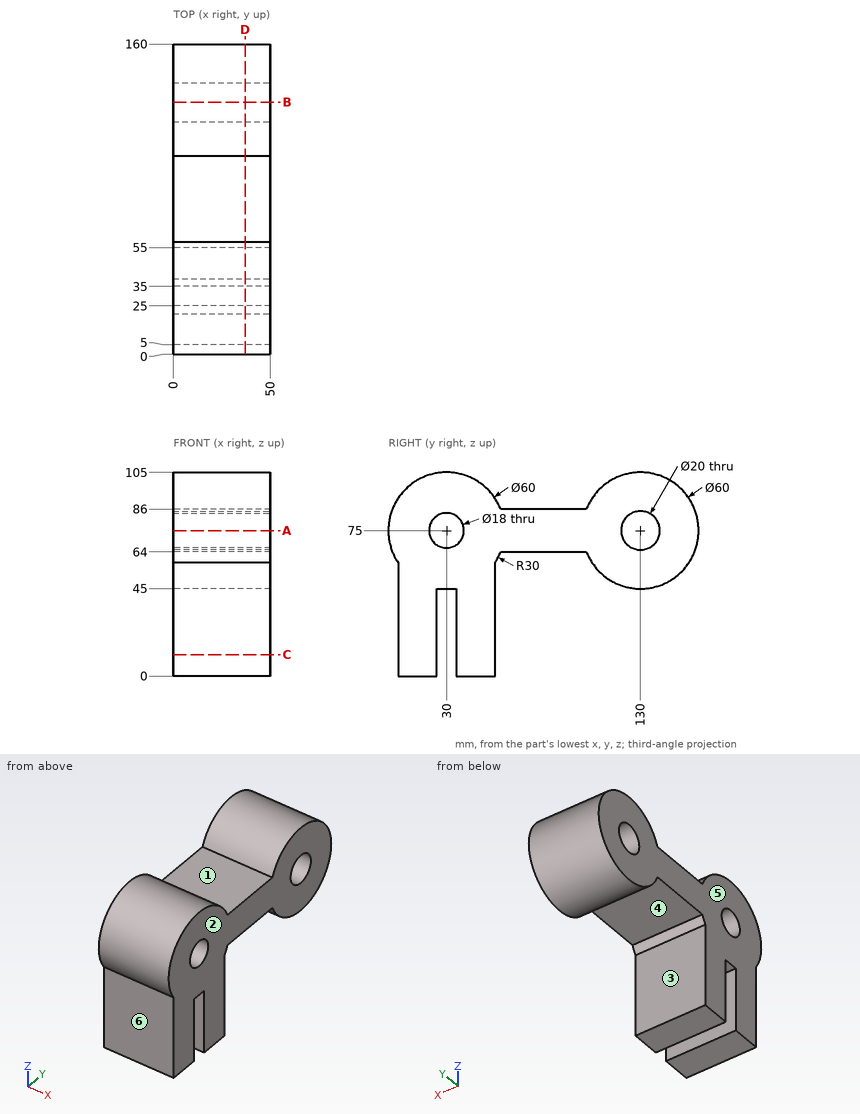
Print and shaded views of the part. All mm, measured from the part's lowest x, y and z. A direction names the side the tool comes from. Coordinates: 2 decimals unless noted, no trailing zeros. Loops run counter-clockwise (first coordinate to the right, second up) from the corner with the lowest first, then second, coordinate; pieces in that order, holes last. Notation, with made-up numbers: (5.5, -37) -> (41.5, -37) arc R24 cw to (41.5, -5) -> close; hole circle Ø6 at (46.5, -32.5). An arc over 180 degrees is marked (long way). Use a Markdown table: item, result. Add a question column.
Item 1: Band-saw the part on B-B on y = 130. Write the cut outline in (x, z).
Item 2: Probe probe 1 along Y at (x, z) = (18.5, 75); probe 2 along Y at (x, z) = (8.5, 41); probe 3 along Y at (x, z) = (46, 97.5). List the from-to ranges inside material, lowest first.
Item 3: Which spindle directions (+Z, -Z, +X, -X, +Y, -Y) get a long thin tool onto all of the face, cutting with end or side? Do the marked faces 1, 2 and 3. Say none if no direction does.
Item 4: Pull direction Y, two halves, no side cores. Call the marked faces 4, 5 and 6: +Y half, -Y half, draft (parallel to the pull), parting line (faces both ways), or undercut.
Item 5: Band-saw the part on A-A on z = 75. Write the cut outline in (x, y).
Item 6: Flat gauge pins, fed straight in: P1, Ø8, axis at y = 26.5, z = 15, coming from the -X side; P2, Ø2, axis at x = 22, y = 127.5, coming from the -Z side; P3, Ø16, axis at y = 30, z = 75, coming from the -X side; P4, Ø3, axis at x = 39, y = 84, coming from the +Z side. Where does each tip first touch, or does it go through?
Item 7: Band-saw the part on C-C on z = 11. Write the cut outline in (x, y), plus the area to 3 significant figures.
Item 8: Band-saw the part on D-D on x = 37. Write the cut outline in (y, z).
Geometry says:
| question | item | result |
|---|---|---|
| 1 | outline | (0, 45) -> (50, 45) -> (50, 65) -> (0, 65) -> close; (0, 85) -> (50, 85) -> (50, 105) -> (0, 105) -> close |
| 2 | probe 1 | 0 to 21, 39 to 120, 140 to 160 |
| 2 | probe 2 | 5 to 25, 35 to 55 |
| 2 | probe 3 | 10.16 to 49.84, 110.16 to 149.84 |
| 3 | face 1 | +Z, +X, -X |
| 3 | face 2 | +Z, -Z, +X, +Y, -Y |
| 3 | face 3 | -Z, +X, -X |
| 4 | face 4 | undercut |
| 4 | face 5 | draft |
| 4 | face 6 | -Y half |
| 5 | outline | (0, 0) -> (50, 0) -> (50, 21) -> (0, 21) -> close; (0, 39) -> (50, 39) -> (50, 120) -> (0, 120) -> close; (0, 140) -> (50, 140) -> (50, 160) -> (0, 160) -> close |
| 6 | P1 | x = 0 |
| 6 | P2 | z = 45.04 |
| 6 | P3 | through |
| 6 | P4 | z = 86 |
| 7 | outline | (0, 5) -> (50, 5) -> (50, 25) -> (0, 25) -> close; (0, 35) -> (50, 35) -> (50, 55) -> (0, 55) -> close |
| 7 | area | 2,000 mm² |
| 8 | outline | (5, 0) -> (25, 0) -> (25, 45) -> (35, 45) -> (35, 0) -> (55, 0) -> (55, 58.42) arc R30 ccw to (57.91, 64) -> (102.09, 64) arc R30 ccw (long way) to (102.09, 86) -> (57.91, 86) arc R30 ccw (long way) to (5, 58.42) -> close; hole circle Ø18 at (30, 75); hole circle Ø20 at (130, 75) |
